Check sheet for the drawn part. Datum: minimum x, y, z corner. Units: mm. A direction names the side the tool comes from. Give positions to 0.01 mm unless a question says otherwise; leave off trailing zeros. Order: outer loops, then holes, each group sorted by start corner. A loop starts at its lowest first (then second) coordinate and runs counter-clockwise, first axis right, second up. Notation, with made-up numbers: (0.25, 53) -> (4.25, 53) arc R12 cw to (4.25, 65) -> close; hole circle Ø11 at (75.25, 27.25). An arc over 180 degrees is marked (long way). Answer in a Markdown table with one row per item. Add a question column.
(1) Thickness scan on L1, parallel to X at y = 46, z = 41; L2, parallel to Y at x = 68.5, z = 66.5; L3, parallel to Z at x = 41, y = 46 (1 decimal). Record the ranges inside material, lowest first. Write a range as [from, to].
(2) Cross-section at C-C (z = 80.5). Record the cut outline in (x, y).
(3) Cross-section at D-D (y = 27.5). Record the cut outline in (x, z) (1 decimal), then the cut area to 3 significant figures.
(4) Release check for a two-part mould opening along X. For the marked faces 4, 5, 6 and 7 record: released by +X, released by -X, zero draft, split by the parting line, or undercut.
(5) Cross-section at A-A (z = 41.5). Record the cut outline in (x, y).
(6) Go/stop test with flat-tipped pins: pin 1 (16 mm diameter, centred on y = 14.5, z = 92.5, fed in from -X); pin 2 (8 mm diameter, centred on x = 25.5, y = 28, fed in from -Z); pin 3 (12 mm diameter, centred on x = 20, y = 32, fed in from -Z) (1 decimal); pin 4 (12 mm diameter, centred on x = 22, z = 119.5, fed in from -Y). Record where each tip stops, or that it passes through.
(7) Cross-section at B-B (x = 41.5). Record the cut outline in (y, z), then the cut area to 3 significant figures.
(8) Set-up check for the marked faces 1, 2 and 3: record each of +Z, -Z, +X, -X, +Y, -Y from which the full face is reachable in a straight line by a thin tool's end or side.
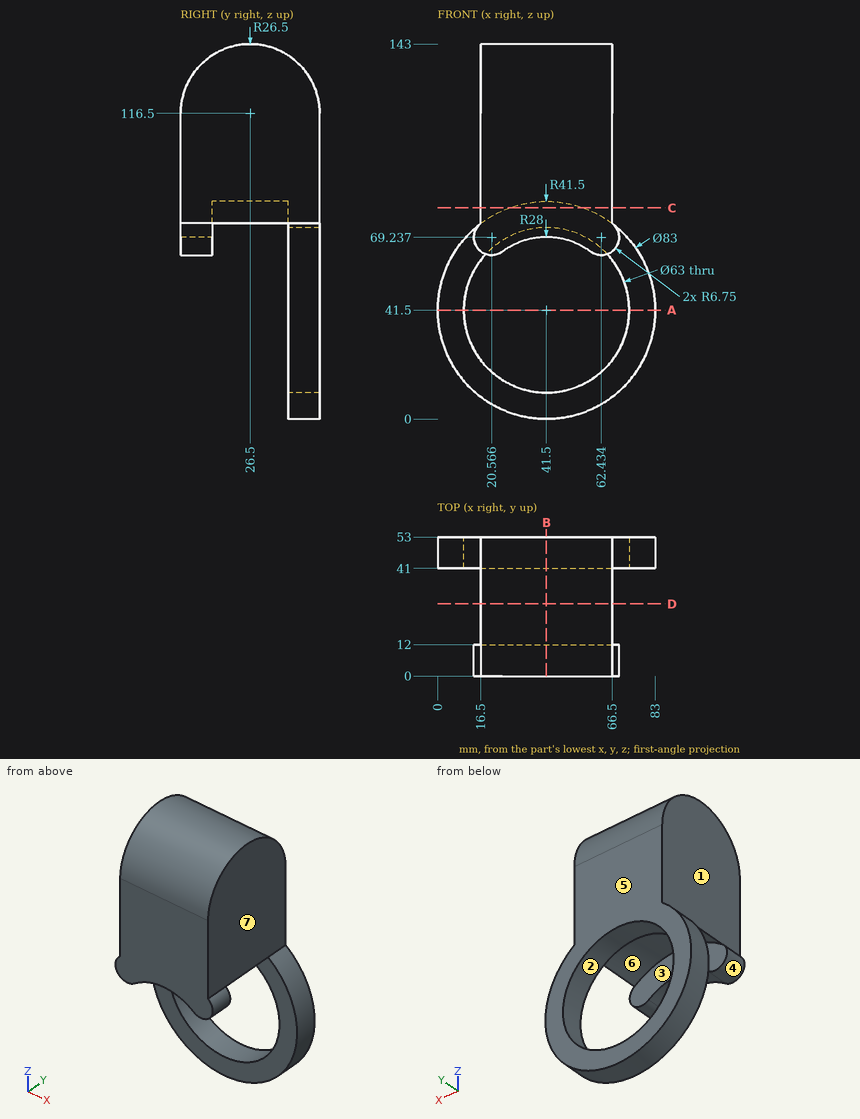
Answer below:
| question | item | result |
|---|---|---|
| 1 | L1 | x = [0, 10], [73, 83] |
| 1 | L2 | y = [0, 12], [41, 53] |
| 1 | L3 | z = [0, 10], [73, 134.4] |
| 2 | outline | (16.5, 0) -> (66.5, 0) -> (66.5, 53) -> (16.5, 53) -> close; hole (27.31, 12) -> (55.69, 12) -> (55.69, 41) -> (27.31, 41) -> close |
| 3 | outline | (16.5, 74.6) arc R41.5 cw to (66.5, 74.6) -> (66.5, 143) -> (16.5, 143) -> close |
| 3 | area | 3,130 mm² |
| 4 | face 4 | undercut |
| 4 | face 5 | zero draft |
| 4 | face 6 | undercut |
| 4 | face 7 | released by +X |
| 5 | outline | (0, 41) -> (10, 41) -> (10, 53) -> (0, 53) -> close; (73, 41) -> (83, 41) -> (83, 53) -> (73, 53) -> close |
| 6 | pin 1 | stops at x = 16.5 |
| 6 | pin 2 | stops at z = 77.86 |
| 6 | pin 3 | stops at z = 74.6 |
| 6 | pin 4 | stops at y = 0 |
| 7 | outline | (0, 69.5) -> (12, 69.5) -> (12, 83) -> (41, 83) -> (41, 73) -> (53, 73) -> (53, 116.5) arc R26.5 ccw to (0, 116.5) -> close; (41, 0) -> (53, 0) -> (53, 10) -> (41, 10) -> close |
| 7 | area | 3,280 mm² |
| 8 | face 1 | +Z, -X, +Y, -Y |
| 8 | face 2 | +Y |
| 8 | face 3 | -Z |
